Here's how the part is built. I have some questions about the finished solid (model axes, mm). A direction names the side the tool comes from. Coordinates: 2 decimals unless noted, no trailing zeros. Write each loop counter-clockwise with the first axis right and the second up, starting at its lowest first coordinate (ties: lowest second). Pieces come first, ordered by that corner, then holes.
Item 1: I want a section at A-A (z = -7). Please give me the cut outline in (x, y).
Item 2: For faces 1 (the face through (13.58, 26.6, -15.82)), 2 (the face through (-0.44, 51.946, 23.335)), 3 (the face through (23.487, 24.75, -12.845)), 4 (the face through (-0.22, 49.05, 31.36)), which set-ups out of +Z, -Z, +X, -X, +Y, -Y let a thin tool reach every point of the face, with its end or its side?
Item 3: I want a section at B-B (x = -18.5). Please give me the cut outline in (y, z).
Item 4: Please list where these lines run through material, in increasing order: line 1 (Y direction, x = 20.5, z = 24); line 2 (X direction, y = 18, z = -12.5); line 3 (Y direction, x = -29, z = 48).
Item 5: I want a section at C-C (y = 16). Please give me the cut outline in (x, z).
Item 6: If we mould it in two halves opening along Y, with no side actions, what happens to faces 5 (the face through (0, -12, -5.663)), 6 (the face through (24.306, 12.466, -7.454)), 7 (the face through (23.08, 27.674, -16.582))? For each: pulls with the +Y half, pulls with the -Y half, needs draft (parallel to the pull), parting line crosses it, or undercut.
Item 7: I'm going to push flat-ended pins straight in: P1, Ø5, axis at x = -23.5, z = 44, coming from the +Y side; P2, Ø15.5, axis at y = 32, z = 40.5, coming from the -X side; P3, Ø4, axis at x = -14, y = -3, coming from the -Z side. Where does each tip first touch, or does it pass through?
Item 8: I want a section at D-D (z = 36). Count the separate pieces of the cut face and the enclosed holes in it, and give its area (3 significant figures).
from build123d import *
from OCP.BRepFilletAPI import BRepFilletAPI_MakeChamfer

# Parameters (mm, degrees)
EXTRUDE_2_DEPTH                 = 37.5
CUT_EXTRUDE_7_DEPTH             = 103.837497834
CUT_EXTRUDE_7_DEPTH_BACK        = 103.837497834
CUT_EXTRUDE_3_DEPTH             = 103.837497834
CUT_EXTRUDE_3_DEPTH_BACK        = 103.837497834
CUT_EXTRUDE_4_REACH             = 108.804
CUT_EXTRUDE_4_DIRECTION_2_DEPTH = 107.803974103
FILLET_1_R                      = 10
FILLET_2_R                      = 10
CHAMFER_1_SIZE                  = 10
CHAMFER_1_SIZE2                 = 7.348769571
CHAMFER_1_SIZE2_2               = 7.320508076
FILLET_4_R                      = 4
FILLET_5_R                      = 4
FILLET_6_R                      = 4
FILLET_7_R                      = 4
FILLET_8_R                      = 4
CUT_EXTRUDE_5_REACH             = 86.613
FILLET_9_R                      = 4
CUT_EXTRUDE_19_DEPTH            = 0.5


with BuildPart() as part:
    # 草图1 → 凸台-拉伸2 (new, symmetric)
    with BuildSketch(Plane(origin=(0, 0, 0), x_dir=(0, 0, -1), z_dir=(1, 0, 0))):
        Polygon((-69.337215993, -13.957199945), (5.662784007, -13.957199945), (5.662784007, -9.457199945), (-62.541106353, -9.457199945), (-37.306862797, 34.249791985), (-22.77752063, 59.415350818), (-6.506208301, 32.121536588), (7.539405244, 8.561152577), (17.593990312, 25.976204763), (15.540885381, 29.420122711), (6.662784007, 14.042800055), (-24.337215993, 66.042800055), align=None)
    extrude(amount=EXTRUDE_2_DEPTH, both=True)

    # 草图3 → 切除-拉伸-薄壁7 (cut, two sides: drawn at the far end of the back side and taken through both)
    with BuildSketch(Plane.XY.offset(-CUT_EXTRUDE_7_DEPTH_BACK)):
        Polygon((-30, 66.042800055), (-37.5, -13.957199945), (-47.456342261, -13.023792858), (-39.956342261, 66.976207142), align=None)
    extrude(amount=CUT_EXTRUDE_7_DEPTH + CUT_EXTRUDE_7_DEPTH_BACK, mode=Mode.SUBTRACT)

    # 草图5 → 切除-拉伸3 (cut, two sides: drawn at the far end of the back side and taken through both)
    with BuildSketch(Plane.XY.offset(-CUT_EXTRUDE_3_DEPTH_BACK)):
        Polygon((37.5, 66.042800055), (37.5, -13.957199945), (30, 66.042800055), align=None)
    extrude(amount=CUT_EXTRUDE_3_DEPTH + CUT_EXTRUDE_3_DEPTH_BACK, mode=Mode.SUBTRACT)

    # 草图7 → 切除-拉伸4 (cut, up to next)
    with BuildSketch(Plane(origin=(0, 6.612698137, -11.092267843), x_dir=(-1, 0, 0), z_dir=(0, 0.5120645423166438, -0.8589469742085631)), mode=Mode.PRIVATE) as cut_extrude_4_sk1:
        Polygon((-10, 28.600496992), (10, 28.600496992), (15, 0), (-15, 0), align=None)
    cut_extrude_4_tool1 = extrude(cut_extrude_4_sk1.sketch, amount=-CUT_EXTRUDE_4_REACH, mode=Mode.PRIVATE) & part.part
    add(cut_extrude_4_tool1.solids().sort_by_distance((0, 18.076976, -4.257794))[0], mode=Mode.SUBTRACT)

    # 草图7 → 切除-拉伸4 direction 2 (cut)
    with BuildSketch(Plane(origin=(0, 6.612698137, -11.092267843), x_dir=(-1, 0, 0), z_dir=(0, 0.5120645423166438, -0.8589469742085631))):
        Polygon((-10, 28.600496992), (10, 28.600496992), (15, 0), (-15, 0), align=None)
    extrude(amount=CUT_EXTRUDE_4_DIRECTION_2_DEPTH, mode=Mode.SUBTRACT)

    # 圆角1
    fillet_1_edges = [part.edges().sort_by_distance(p)[0] for p in [
        (37.2890625, -11.707199945, -5.662784007),
    ]]
    fillet(fillet_1_edges, radius=FILLET_1_R)

    # 圆角2
    fillet_2_edges = [part.edges().sort_by_distance(p)[0] for p in [
        (-37.2890625, -11.707199945, -5.662784007),
    ]]
    fillet(fillet_2_edges, radius=FILLET_2_R)

    # 倒角1: one chamfer whose edges measure the first distance from different faces: ONE call of the kernel's chamfer builder (chamfer() names one face for all edges)
    chamfer_1_edges_1 = [part.edges().sort_by_distance(p)[0] for p in [
        (0, 59.415350818, 22.77752063),
    ]]
    chamfer_1_side_1 = [part.faces().sort_by_distance(p)[0] for p in [
        (0, 23.884294487, 43.291385568),
    ]]
    chamfer_1_edges_2 = [part.edges().sort_by_distance(p)[0] for p in [
        (0, -9.457199945, 62.541106353),
    ]]
    chamfer_1_side_2 = [part.faces().sort_by_distance(p)[0] for p in [
        (0, -9.457199945, 28.713118307),
    ]]
    chamfer_1 = BRepFilletAPI_MakeChamfer(part.part.solid().wrapped)
    for e in chamfer_1_edges_1:
        chamfer_1.Add(CHAMFER_1_SIZE, CHAMFER_1_SIZE2, e.wrapped, chamfer_1_side_1[0].wrapped)  # the first distance lies on this face
    for e in chamfer_1_edges_2:
        chamfer_1.Add(CHAMFER_1_SIZE, CHAMFER_1_SIZE2_2, e.wrapped, chamfer_1_side_2[0].wrapped)  # the first distance lies on this face
    add(Compound.cast(chamfer_1.Shape()), mode=Mode.REPLACE)

    # 圆角4
    fillet_4_edges = [part.edges().sort_by_distance(p)[0] for p in [
        (0, -13.957199945, 69.337215993),
    ]]
    fillet(fillet_4_edges, radius=FILLET_4_R)

    # 圆角5
    fillet_5_edges = [part.edges().sort_by_distance(p)[0] for p in [
        (0, 66.042800055, 24.337215993),
    ]]
    fillet(fillet_5_edges, radius=FILLET_5_R)

    # 圆角6
    fillet_6_edges = [part.edges().sort_by_distance(p)[0] for p in [
        (24.181372827, 14.042800055, -6.662784007),
        (-24.181372827, 14.042800055, -6.662784007),
    ]]
    fillet(fillet_6_edges, radius=FILLET_6_R)

    # 圆角7
    fillet_7_edges = [part.edges().sort_by_distance(p)[0] for p in [
        (24.88913288, 8.561152577, -7.539405244),
        (-24.88913288, 8.561152577, -7.539405244),
    ]]
    fillet(fillet_7_edges, radius=FILLET_7_R)

    # 圆角8
    fillet_8_edges = [part.edges().sort_by_distance(p)[0] for p in [
        (12.323882788, 27.698163737, -16.567437846),
        (-12.323882788, 27.698163737, -16.567437846),
        (-33.594809655, 27.698163737, -16.567437846),
        (33.594809655, 27.698163737, -16.567437846),
    ]]
    fillet(fillet_8_edges, radius=FILLET_8_R)

    # 切除-拉伸5: up to this plane
    cut_extrude_5_end = Plane(origin=(37.5, 34.249791985, 37.306862797), z_dir=(0, 0.5000000000000044, 0.8660254037844362))
    # 草图8 → 切除-拉伸5 (cut, up to the surface)
    with BuildSketch(Plane(origin=(0, 26.273073909, 46.70768695), x_dir=(1, 0, 0), z_dir=(0, 0.4902612396325587, 0.8715755371245495)), mode=Mode.PRIVATE) as cut_extrude_5_sk1:
        with BuildLine():
            Line((9.862156139, 17.515327615), (9.862156139, -14.832544522))
            ThreePointArc((9.862156139, -14.832544522), (0, -24.694700661), (-9.862156139, -14.832544522))
            Line((-9.862156139, -14.832544522), (-9.862156139, 17.515327615))
            ThreePointArc((-9.862156139, 17.515327615), (0, 27.377483754), (9.862156139, 17.515327615))
        make_face()
    cut_extrude_5_tool1 = split(extrude(cut_extrude_5_sk1.sketch, amount=-CUT_EXTRUDE_5_REACH, mode=Mode.PRIVATE), bisect_by=cut_extrude_5_end, keep=Keep.BOTH, mode=Mode.PRIVATE)
    add(cut_extrude_5_tool1.solids().sort_by_distance((0, 27.442198, 46.050055))[0], mode=Mode.SUBTRACT)

    # 圆角9
    fillet_9_edges = [part.edges().sort_by_distance(p)[0] for p in [
        (10, 30.653121751, 4.435165153),
        (-10, 30.653121751, 4.435165153),
    ]]
    fillet(fillet_9_edges, radius=FILLET_9_R)

    # 草图9 → 切除-拉伸19 (cut)
    # profile 1 of 2: a face of its own
    with BuildSketch(Plane(origin=(0, 6.612698137, -11.092267843), x_dir=(-1, 0, 0), z_dir=(0, 0.5120645423166438, -0.8589469742085631))):
        with BuildLine():
            add(Edge.make_bspline(
                [(-6.606037662, 38.953429024), (-5.711334874, 40.311243339), (-3.854311729, 43.564154073), (-0.858400361, 45.826493842), (0.468870754, 47.38516919)],
                knots=[0, 0, 0, 0, 0.444342779, 1, 1, 1, 1], degree=3))
            add(Edge.make_bspline(
                [(-6.606037662, 38.953429024), (-9.378559135, 35.780697287), (-14.751433674, 24.057721204), (-5.055372805, 30.986280975)],
                knots=[0, 0, 0, 0, 0.897758924, 0.897758924, 0.897758924, 0.897758924], degree=3))
            add(Edge.make_bspline(
                [(-5.055372805, 30.986280975), (-3.951139058, 31.775338472), (-2.651465095, 32.806301591), (-1.130252381, 34.119348895)],
                knots=[0.897758924, 0.897758924, 0.897758924, 0.897758924, 1, 1, 1, 1], degree=3))
            add(Edge.make_bspline(
                [(6.332322248, 42.490883232), (6.421345736, 41.744828612), (6.344182877, 40.360506044), (6.000591752, 38.579631764), (5.252680808, 37.443200943), (4.475701743, 36.345853392), (3.207138679, 35.357882181), (1.705465876, 34.34846817), (0.163062797, 33.924083238), (-0.754774414, 34.050408523), (-1.130252381, 34.119348895)],
                knots=[0, 0, 0, 0, 0.117072849, 0.219314974, 0.278544439, 0.329333286, 0.430146269, 0.52813716, 0.613566108, 0.673160343, 0.673160343, 0.673160343, 0.673160343], degree=3))
            add(Edge.make_bspline(
                [(0.468870754, 47.38516919), (1.233033198, 47.922620622), (2.49626224, 49.235976382), (4.241552698, 50.722199927), (5.757086701, 51.611825239), (6.890776807, 52.349356015), (7.979867228, 52.911105038), (9.009325049, 52.897932667), (9.772550935, 52.701828247), (10.268614434, 51.887019071), (10.101877149, 50.633458002), (9.70577606, 48.904902538), (8.623104825, 46.001853987), (7.426413078, 43.809596625), (6.332322248, 42.490883232)],
                knots=[0, 0, 0, 0, 0.125072756, 0.245842542, 0.307491057, 0.361289695, 0.429653226, 0.46668336, 0.499065273, 0.530480343, 0.584936423, 0.663141117, 0.772009703, 1, 1, 1, 1], degree=3))
        make_face()
        with BuildLine():
            add(Edge.make_bspline(
                [(-5.925793934, 36.893896271), (-6.314452071, 36.418621882), (-10.90174323, 28.38229129), (-2.668424669, 33.749192184), (-2.77783358, 34.475014711)],
                knots=[0, 0, 0, 0, 0.486390134, 1, 1, 1, 1], degree=3))
            add(Edge.make_bspline(
                [(-2.77783358, 34.475014711), (-2.957051517, 34.52370524), (-3.778444373, 34.774634797), (-5.022215854, 35.454494355), (-5.730155434, 36.410802759), (-5.925793934, 36.893896271)],
                knots=[0.761269827, 0.761269827, 0.761269827, 0.761269827, 0.790511254, 0.896348436, 0.975855606, 0.975855606, 0.975855606, 0.975855606], degree=3))
        make_face(mode=Mode.SUBTRACT)
        with BuildLine():
            add(Edge.make_bspline(
                [(-5.704606663, 37.354305889), (-4.82005562, 39.114963546), (-2.167848058, 42.452443751), (1.487716627, 44.915381127), (3.771169156, 45.300026951)],
                knots=[0.035918318, 0.035918318, 0.035918318, 0.035918318, 0.452487374, 0.939525842, 0.939525842, 0.939525842, 0.939525842], degree=3))
            add(Edge.make_bspline(
                [(-5.704606663, 37.354305889), (-4.903172884, 35.848608285), (-2.06778183, 33.826601764), (2.360384852, 34.966954875), (4.576007986, 37.506203367), (6.220363831, 40.221899193), (5.250367062, 43.052302972), (4.513305616, 44.655132724), (3.771169156, 45.300026951)],
                knots=[0, 0, 0, 0, 0.248218278, 0.43884002, 0.59987409, 0.733439298, 0.868620911, 1, 1, 1, 1], degree=3))
        make_face(mode=Mode.SUBTRACT)
    # profile 2 of 2: a face of its own
    with BuildSketch(Plane(origin=(0, 6.612698137, -11.092267843), x_dir=(-1, 0, 0), z_dir=(0, 0.5120645423166438, -0.8589469742085631))):
        with BuildLine():
            add(Edge.make_bspline(
                [(-6.606037662, 38.953429024), (-6.857731684, 39.967243119), (-6.66251098, 41.958089443), (-5.736175757, 44.327135585), (-4.335162577, 45.931678579), (-2.409061861, 47.170333165), (-0.663837917, 47.683486872), (0.468870754, 47.38516919)],
                knots=[0, 0, 0, 0, 0.241647458, 0.464965071, 0.586300838, 0.737202049, 1, 1, 1, 1], degree=3))
            add(Edge.make_bspline(
                [(-6.606037662, 38.953429024), (-5.711334874, 40.311243339), (-3.854311729, 43.564154073), (-0.858400361, 45.826493842), (0.468870754, 47.38516919)],
                knots=[0, 0, 0, 0, 0.444342779, 1, 1, 1, 1], degree=3))
        make_face()
    extrude(amount=-CUT_EXTRUDE_19_DEPTH, mode=Mode.SUBTRACT)


solid = part.part
Answer:
1. outline: (-35.02, 12.49) - (-13.75, 12.49) - (-12.93, 17.97) - (-34.51, 17.97) - close; (12.93, 17.97) - (13.75, 12.49) - (35.02, 12.49) - (34.51, 17.97) - close
2. face 1: -Z
2. face 2: +X, -X
2. face 3: +X, -X, +Y
2. face 4: +Z
3. outline: (-13.96, -5.66) - (-9.46, -5.66) - (-9.46, 52.54) - (-3.12, 58.88) - (50.76, 27.78) - (53.1, 19.01) - (14.42, -4.05) arc R4 ccw to (14.47, -10.95) - (25.98, -17.59) - (29.42, -15.54) - (19.95, -10.07) arc R4 cw to (19.9, -3.17) - (60.11, 20.8) arc R4 ccw to (60.02, 27.72) - (-8, 65.98) arc R4 ccw to (-13.96, 62.5) - close
4. line 1: y = -13.96 to -9.46, 51.77 to 62.06
4. line 2: x = -34.5 to -13.42, 13.42 to 34.5
4. line 3: y = -13.96 to -9.46, 15.73 to 23.98
5. outline: (-34.69, -11.83) - (-13.66, -11.83) - (-12.88, -3.1) - (-34.69, -3.1) - close; (-34.69, 47.84) - (-9.86, 47.84) - (-9.86, 52.49) - (-34.69, 52.49) - close; (9.86, 47.84) - (34.69, 47.84) - (34.69, 52.49) - (9.86, 52.49) - close; (12.88, -3.1) - (13.66, -11.83) - (34.69, -11.83) - (34.69, -3.1) - close
6. face 5: needs draft
6. face 6: undercut
6. face 7: pulls with the +Y half
7. P1: stops at y = 35.53
7. P2: stops at x = -33.88
7. P3: stops at z = 57
8. separate pieces: 3
8. enclosed holes: 0
8. area: 735 mm2
